The listing builds one solid part. Answer for the finished solid, in the listing's coordinates (mm). Coordinates: 2 decimals unless noted, no trailing zeros. Order: outer loops, then holes, each group sorted by start corner. A loop starts at its lowest first (then second) coordinate and runs counter-clockwise, first axis right, second up. Notation, with made-up numbers: (30.5, 23.25) -> (75.5, 23.25) arc R19 cw to (75.5, 52.25) -> close; hole circle Ø8 at (3.25, 8). An arc over 180 degrees is marked (long way). Return JSON: item names as keys, results as strings.
from build123d import *

# Parameters (mm, degrees)
SKETCH1_W                       = 12.5
SKETCH1_H                       = 220
BLOCO_DEPTH                     = 20.4
REBAIXO_M6_PASSANTE_D           = 6.6
REBAIXO_M6_PASSANTE_CBORE_D     = 11
REBAIXO_M6_PASSANTE_CBORE_DEPTH = 6
FURO_M5X0_8_PASSANTE_D          = 4.2


with BuildPart() as part:
    # Sketch1 → Bloco (new body)
    with BuildSketch(Plane(origin=(0, 0, 0), x_dir=(1, 0, 0), z_dir=(0, 1, 0))):
        with Locations((6.25, 110)):
            Rectangle(SKETCH1_W, SKETCH1_H)
    extrude(amount=BLOCO_DEPTH)

    # Rebaixo M6 - Passante (through all)
    with Locations(Plane(origin=(0, 20.4, 0), x_dir=(1, 0, 0), z_dir=(0, 1, 0))):
        with Locations((6.25, 10), (6.25, 110), (6.25, 210)):
            CounterBoreHole(REBAIXO_M6_PASSANTE_D / 2, REBAIXO_M6_PASSANTE_CBORE_D / 2, REBAIXO_M6_PASSANTE_CBORE_DEPTH)

    # Furo M5x0.8 - Passante (through all)
    with Locations(Plane(origin=(0, 20.4, 0), x_dir=(1, 0, 0), z_dir=(0, 1, 0))):
        with Locations((6.25, 50), (6.25, 170)):
            Hole(FURO_M5X0_8_PASSANTE_D / 2)


solid = part.part
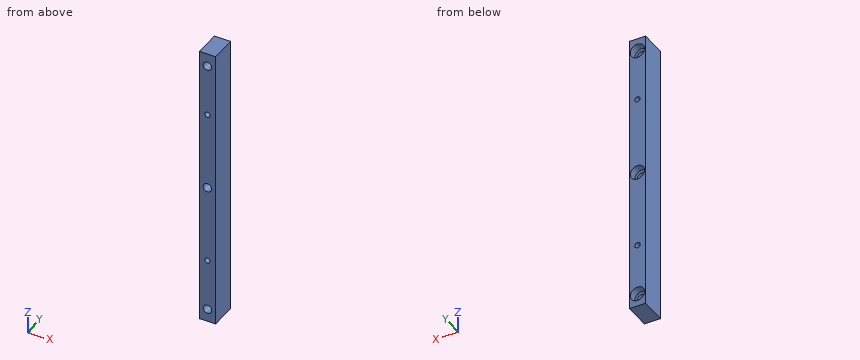
1. The part is cut by section D-D on z = -50. Give the vertices of the cut face in (x, y), and give its area (3 significant figures).
Answer block:
{"outline": "(0, 0) -> (4.15, 0) -> (4.15, 20.4) -> (0, 20.4) -> close; (8.35, 0) -> (12.5, 0) -> (12.5, 20.4) -> (8.35, 20.4) -> close", "area": "169 mm2"}
2. Consider line 1 (Z direction, x = 6.25, y = 5.75); line 2 (X direction, y = 17.85, z = -210); line 3 (Z direction, x = 4, y = 9.25). Determine where each line is inside the solid, lowest interval first. Write a range as from..to.
Answer block:
{"line 1": "z = -220..-213.3, -206.7..-172.1, -167.9..-113.3, -106.7..-52.1, -47.9..-13.3, -6.7..0", "line 2": "x = 0..0.75, 11.75..12.5", "line 3": "z = -220..-212.41, -207.59..-112.41, -107.59..-12.41, -7.59..0"}
3. Each of these flat-tipped pins is pushed along its axis until it touches: pin 1 Ø5.5 at (x, z) = (6.25, -10) entering from -Y; pin 2 Ø4 at (x, z) = (3, -196.5) entering from -Y; pin 3 Ø7.5 at (x, z) = (6.25, -210) entering from +Y. Where does it stop, or does it pass through?
Answer block:
{"pin 1": "passes through", "pin 2": "stops at y = 0", "pin 3": "stops at y = 14.4"}
4. The part is cut by section B-B on y = 16.5. Give the vertices of the cut face in (x, z), and give its area (3 significant figures).
Answer block:
{"outline": "(0, -220) -> (12.5, -220) -> (12.5, 0) -> (0, 0) -> close; hole circle Ø11 at (6.25, -210); hole circle Ø11 at (6.25, -110); hole circle Ø11 at (6.25, -10); hole circle Ø4.2 at (6.25, -170); hole circle Ø4.2 at (6.25, -50)", "area": "2,440 mm2"}
5. The part is cut by section A-A on z = -110. Give the vertices of the cut face in (x, y), and give its area (3 significant figures).
Answer block:
{"outline": "(0, 0) -> (2.95, 0) -> (2.95, 14.4) -> (0.75, 14.4) -> (0.75, 20.4) -> (0, 20.4) -> close; (9.55, 0) -> (12.5, 0) -> (12.5, 20.4) -> (11.75, 20.4) -> (11.75, 14.4) -> (9.55, 14.4) -> close", "area": "94.0 mm2"}
6. The part is cut by section C-C on x = 6.25. Give the number of separate pieces and of enclosed holes in the cut face, and give its area (3 significant figures).
Answer block:
{"separate pieces": "6", "enclosed holes": "0", "area": "3,830 mm2"}
